from build123d import *

# Parameters (mm, degrees)
F0_W     = 100
F0_H     = 100
F1_DEPTH = 100
F2_R     = 47.40298
F3_DEPTH = 70
F4_R     = 47.561865
F5_DEPTH = 70
F6_R     = 35
F7_DEPTH = 47.562865


with BuildPart() as f1:
    # F0 (on Front) → F1 (new body)
    with BuildSketch(Plane.XZ):
        with Locations((50, 50)):
            Rectangle(F0_W, F0_H)
    extrude(amount=F1_DEPTH)

    # F2 (on Top) → F3 (join)
    with BuildSketch(Plane.XY):
        Circle(F2_R)
    extrude(amount=F3_DEPTH)

    # F4 (on Top) → F5 (join)
    with BuildSketch(Plane.XY):
        Circle(F4_R)
    extrude(amount=F5_DEPTH)

    # F6 (on Right) → F7 (cut, through all)
    with BuildSketch(Plane.YZ):
        with Locations((0, 58.089419)):
            Circle(F6_R)
    extrude(amount=-F7_DEPTH, mode=Mode.SUBTRACT)


solid = f1.part
Geometry check sheet. Reference: the model listing, model coordinates, mm. A direction names the side the tool comes from. Give positions to 0.01 mm unless a question says otherwise; leave off trailing zeros. Write each loop counter-clockwise with the first axis right and the second up, starting at its lowest first coordinate (ties: lowest second). Pieces come first, ordered by that corner, then holes.
1) Release check for a two-part mould opening along Z. For faces 5 (the face through (49, -100, 51)), 6 (the face through (-18.2, -0.9, 23.1)), 7 (the face through (49, -49, 100)) record: released by +Z, released by -Z, zero draft, split by the parting line, or undercut.
Values follow:
face 5: zero draft
face 6: undercut
face 7: released by +Z
2) Thickness scan on line 1 (Z direction, x = -16, y = 0); line 2 (X direction, y = -48, z = 93); line 3 (Y direction, x = 49, z = 77). Record the ranges inside material, lowest first.
Values follow:
line 1: z = 0 to 23.09
line 2: x = 0 to 100
line 3: y = -100 to 0
3) Cross-section at A-A (z = 66.5). Record the boundary of the cut face in (x, y), plus the area to 3 significant figures.
Values follow:
outline: (-33.28, -33.97) arc R47.56 ccw to (0, -47.56) - (0, -100) - (100, -100) - (100, 0) - (47.56, 0) arc R47.56 ccw to (-33.28, 33.97) - (0, 33.97) - (0, -33.97) - close
area: 12,400 mm2
4) Go/stop test with flat-tipped pins: pin 1 Ø1 at (y, z) = (-33.5, 68.5) entering from -X; pin 2 Ø4 at (x, z) = (-13.5, 24.5) entering from +Y; pin 3 Ø1.5 at (y, z) = (-32, 85.5) entering from -X. Record where each tip stops, or that it passes through.
Values follow:
pin 1: stops at x = -33.99
pin 2: stops at y = 46.15
pin 3: stops at x = 0
5) Cross-section at D-D (z = 53). Record the boundary of the cut face in (x, y).
Values follow:
outline: (-32.6, -34.63) arc R47.56 ccw to (0, -47.56) - (0, -100) - (100, -100) - (100, 0) - (47.56, 0) arc R47.56 ccw to (-32.6, 34.63) - (0, 34.63) - (0, -34.63) - close
6) Cross-section at C-C (x = 62). Record the boundary of the cut face in (y, z).
Values follow:
outline: (-100, 0) - (0, 0) - (0, 100) - (-100, 100) - close
7) Cross-section at B-B (y = -83). Record the boundary of the cut face in (x, z), plus the area to 3 significant figures.
Values follow:
outline: (0, 0) - (100, 0) - (100, 100) - (0, 100) - close
area: 10,000 mm2
8) Set-up check for faces 1 (the face through (100, -49, 49)), 2 (the face through (-14, -39, 70)), 3 (the face through (15, 24, 70)), 4 (the face through (60, 0, 62)): record each of +Z, -Z, +X, -X, +Y, -Y from which the full face is reachable in a straight line by a thin tool's end or side.
Values follow:
face 1: +Z, -Z, +X, +Y, -Y
face 2: +Z, -X, +Y, -Y
face 3: +Z, +X, -X, +Y
face 4: +Z, +X, +Y
